Geometry: see drawing. Coordinates: mm, zero at the bounding-box minimum. A direction names the side the tool comes from. Round coordinates to 2 decimals unless told otherwise and drop trailing zeros. Loops run counter-clockwise (first coordinate to the right, second up) from the corner with the lowest first, then second, coordinate; pieces in that order, holes last.
(1) Cut plane D-D, the plane z = 59. Output: boundary loops of the cut face in (x, y).
(2) Draft query along Z for the marked faces 1, 2 and 3. Return one class per face: released by +Z, released by -Z, zero draft, split by the parting line, or undercut.
(3) Cut plane B-B, the plane x = 46. Output: boundary loops of the cut face in (y, z).
(4) First-contact query: pin 1 Ø4 at (y, z) = (3, 78) entering from -X; pin 2 Ø1.5 at (x, y) = (119, 2.5) entering from -Z. Flat tips, straight axial feed; report the tip coordinate or a pass-through.
(5) Cut plane C-C, the plane x = 169.5. Output: boundary loops of the cut face in (y, z), and give its area (3 significant figures).
(6) Access query for the marked faces 4, 5 and 6. Directions: +Z, -Z, +X, -X, +Y, -Y. A direction counts if a zero-diameter tool reaches every point of the face in a straight line with its end or side. Return the directions, or none.
(7) Line query: line 1 (Z direction, x = 103, y = 39); line 2 (Y direction, x = 150, z = 85.5); line 3 (Z direction, x = 39.5, y = 14). Output: solid intervals per line, ascending.
(8) Cut plane A-A, the plane z = 80. Output: boundary loops of the cut face in (x, y).
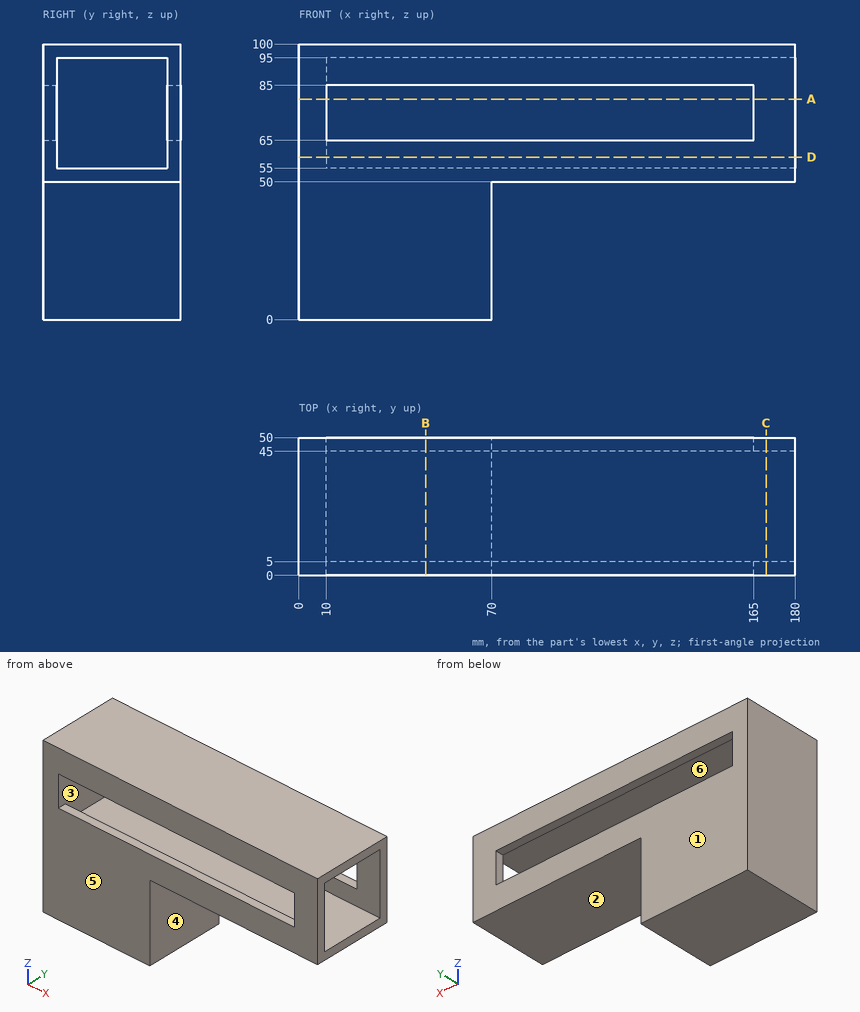
Reported:
1. outline: (0, 0) - (180, 0) - (180, 5) - (10, 5) - (10, 45) - (180, 45) - (180, 50) - (0, 50) - close
2. face 1: zero draft
2. face 2: released by -Z
2. face 3: undercut
3. outline: (0, 0) - (50, 0) - (50, 65) - (45, 65) - (45, 55) - (5, 55) - (5, 65) - (0, 65) - close; (0, 85) - (5, 85) - (5, 95) - (45, 95) - (45, 85) - (50, 85) - (50, 100) - (0, 100) - close
4. pin 1: stops at x = 0
4. pin 2: stops at z = 50
5. outline: (0, 50) - (50, 50) - (50, 100) - (0, 100) - close; hole (5, 55) - (45, 55) - (45, 95) - (5, 95) - close
5. area: 900 mm2
6. face 4: -Z, +X, +Y, -Y
6. face 5: +Z, -Z, +X, -X, -Y
6. face 6: +X
7. line 1: z = 50 to 55, 95 to 100
7. line 2: y = 0 to 5, 45 to 50
7. line 3: z = 0 to 55, 95 to 100
8. outline: (0, 0) - (10, 0) - (10, 50) - (0, 50) - close; (165, 0) - (180, 0) - (180, 5) - (165, 5) - close; (165, 45) - (180, 45) - (180, 50) - (165, 50) - close
